Check sheet for the modelled part. Datum: model origin and axes. Units: mm. Give positions to 0.01 mm unless a question says otherwise; leave off trailing zeros. Loops run counter-clockwise (first coordinate to the right, second up) from the corner with the lowest first, then second, coordinate; pieces in that order, holes last. Notation, with made-up numbers: (39, 48) -> (78, 48) arc R20 ccw to (78, 63) -> close; hole circle Ø11 at (25.25, -25.75). An arc over 180 degrees is marked (long way). Answer as CSV lines item,"result". Start each with the question number.
(1) Material ranges on line 1 (Y direction, x = 0, z = 22.75); line 2 (X direction, y = 16, z = 22.5); line 3 (Y direction, x = -7, z = 16) (3 decimals), recorded low to high. Write a range as from..to.
(2) Section check D-D on x = -17. Enter the section's corners in (y, z).
(3) Section check B-B on z = 7. Enter the section's corners in (x, y), plus the area to 3 significant figures.
(4) Section check C-C on y = -7.5. Enter the section's corners in (x, z), plus the area to 3 significant figures.
(5) Section check A-A on z = 21. Enter the section's corners in (x, y), plus the area to 3 significant figures.
(6) Gauge pin test, flat ends, axial feed: pin 1 Ø1 at (x, z) = (14, 16.5) entering from -Y; pin 2 Ø5 at (y, z) = (-14.5, 6) entering from +X; pin 3 Ø4 at (x, z) = (-6.5, 11) entering from -Y. Record the tip position at first contact, or that the pin passes through.
Autodesk Inventor part; units mm, degrees
ref_plane "YZ Plane" through (0, 0, 0) normal (1, 0, 0) x (0, 1, 0)
ref_plane "XZ Plane" through (0, 0, 0) normal (0, 1, 0) x (-1, 0, 0)
ref_plane "XY Plane" through (0, 0, 0) normal (0, 0, 1) x (1, 0, 0)
sketch "Sketch1" plane through (0, 0, 0) normal (0, 0, 1) x (1, 0, 0)
  circle A0 centre (0, 0) radius 20
  dimension "d0" = 40
extrude "Extrusion1" add sketch "Sketch1" along normal blind 27.1
sketch "Sketch2" plane through (0, 0, 27.1) normal (0, 0, 1) x (1, 0, 0)
  point P0 (0, 0)
  point P1 (0, 0)
hole "Hole1" at (0, 0, 27.1) direction (0, 0, -1) diameter 3.242 depth 8 tip angle 118
chamfer "Chamfer1" distance 0.7 angle 45 1 edges at (0, 1.621, 27.1)
properties part number "CounterWeights_Brass" material "Brass, Soft Yellow"
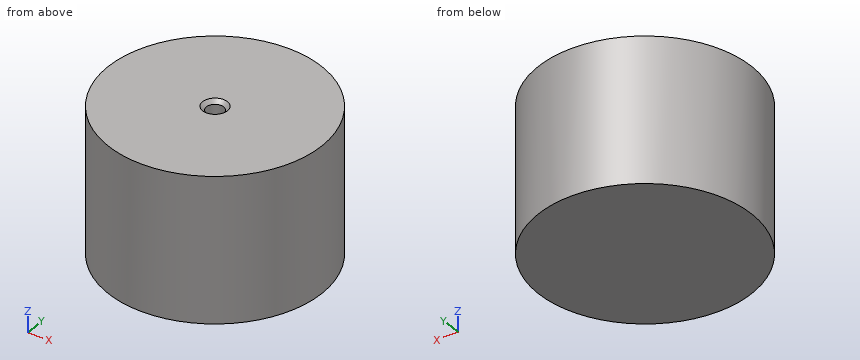
Working result:
1,line 1,"y = -20..-1.62, 1.62..20"
1,line 2,"x = -12..12"
1,line 3,"y = -18.735..18.735"
2,outline,"(-10.54, 0) -> (10.54, 0) -> (10.54, 27.1) -> (-10.54, 27.1) -> close"
3,outline,"circle Ø40 at (0, 0)"
3,area,"1,260 mm^2"
4,outline,"(-18.54, 0) -> (18.54, 0) -> (18.54, 27.1) -> (-18.54, 27.1) -> close"
4,area,"1,000 mm^2"
5,outline,"circle Ø40 at (0, 0); hole circle Ø3.24 at (0, 0)"
5,area,"1,250 mm^2"
6,pin 1,"stops at y = -14.76"
6,pin 2,"stops at x = 16"
6,pin 3,"stops at y = -19.49"
